The listing builds one solid part. Answer for the finished solid, in the listing's coordinates (mm). Coordinates: 2 decimals unless noted, no trailing zeros. Use one line per item in the form item = value. Start each with the question number.
```python
from build123d import *

# Parameters (mm, degrees)
SKETCH1_R           = 6.11
SKETCH1_R_2         = 5
BOSS_EXTRUDE1_DEPTH = 7
CUT_EXTRUDE2_DEPTH  = 7
CIRPATTERN1_COUNT   = 21


with BuildPart() as part:
    # Sketch1 → Boss-Extrude1 (new body)
    with BuildSketch(Plane(origin=(0, 0, 0), x_dir=(1, 0, 0), z_dir=(0, 1, 0))):
        Circle(SKETCH1_R)
        Circle(SKETCH1_R_2, mode=Mode.SUBTRACT)
    extrude(amount=BOSS_EXTRUDE1_DEPTH)

    # Sketch2 → Cut-Extrude2 (cut)
    with BuildSketch(Plane(origin=(0, 0, 0), x_dir=(1, 0, 0), z_dir=(0, 1, 0))):
        with BuildLine():
            Line((0.634953715, -5.878485528), (0.265979235, -5.171237446))
            ThreePointArc((0.265979235, -5.171237446), (0, -5.01), (-0.265979235, -5.171237446))
            Line((-0.265979235, -5.171237446), (-0.634953715, -5.878485528))
            ThreePointArc((-0.634953715, -5.878485528), (-0.765837658, -6.007583501), (-0.947452724, -6.036094212))
            ThreePointArc((-0.947452724, -6.036094212), (0, -7.060330853), (0.947452724, -6.036094212))
            ThreePointArc((0.947452724, -6.036094212), (0.765837658, -6.007583501), (0.634953715, -5.878485528))
        make_face()
    cut_extrude2 = extrude(amount=CUT_EXTRUDE2_DEPTH, mode=Mode.SUBTRACT)

    # CirPattern1: Cut-Extrude2 ×21 about axis
    cirpattern1_axis = Axis((0, 0, 0), (0, 1, 0))
    for i in range(1, CIRPATTERN1_COUNT):
        add(cut_extrude2.rotate(cirpattern1_axis, i * 360 / CIRPATTERN1_COUNT), mode=Mode.SUBTRACT)


solid = part.part
```
(1) Determine the mould class of faces 1 (the face through (-1.08, 3.45, 4.88)), 2 (the face through (-5, 0, -2)) for opening direction Z: +Z half, -Z half, draft (parallel to the pull), parting line (faces both ways), or undercut.
(2) Each of these flat-tipped pins is pushed along its axis until it touches: pin 1 Ø4 at (x, z) = (2, -4.5) entering from -Y; pin 2 Ø1.5 at (y, z) = (3.5, -4) entering from -X. Where does it stop, or does it pass through?
(3) Find the intervals of material crossed by probe 1 along Z at (x, y) = (4.5, 0.5); probe 2 along X at (y, z) = (6.25, 3.5); probe 3 along X at (y, z) = (5, 0), in increasing order. Write a range as from..to.
Evaluation:
q1.face_1 = undercut
q1.face_2 = draft
q2.pin_1 = 0
q2.pin_2 = -4.82
q3.probe_1 = -3.89..-3.06, -2.37..-2.18, 2.18..3.07
q3.probe_2 = -3.91..-3.57, 3.57..3.91
q3.probe_3 = -5.46..-5, 5..5.46
